Autodesk Fusion 360 part; units mm, degrees
sketch "Sketch1" plane through (0, 0, 0) normal (0, 0, 1) x (1, 0, 0)
  line L0 (-26.35, 10.5) -> (-26.35, -10.5)
  line L1 (-26.35, -10.5) -> (-16.35, -10.5)
  line L2 (-16.35, -10.5) -> (-16.35, 10.5)
  line L3 (-16.35, 10.5) -> (16.35, 10.5)
  line L4 (16.35, 10.5) -> (16.35, -10.5)
  line L5 (16.35, -10.5) -> (26.35, -10.5)
  line L6 (26.35, -10.5) -> (26.35, 10.5)
  line L7 (-26.35, -10.5) -> (26.35, 10.5) construction
  line L8 (-26.35, 10.5) -> (-26.35, 31)
  line L9 (-26.35, 31) -> (26.35, 31)
  line L10 (26.35, 31) -> (26.35, 10.5)
  line L11 (-22.75, 31) -> (22.75, 31) construction
  line L12 (22.75, 31) -> (22.75, 10.5) construction
  line L13 (22.75, 10.5) -> (-22.75, 10.5) construction
  line L14 (-22.75, 10.5) -> (-22.75, 31) construction
  line L15 (-22.75, 10.5) -> (22.75, 31) construction
  circle A0 centre (-21.35, 11.9) radius 0.975
  line L16 (-22.75, 20.75) -> (22.75, 20.75) construction
  line L17 (0, 10.5) -> (0, 31) construction
  circle A1 centre (-21.35, 29.6) radius 0.975
  circle A2 centre (21.35, 11.9) radius 0.975
  circle A3 centre (21.35, 29.6) radius 0.975
  circle A4 centre (-12.75, 20.75) radius 8.05
  circle A5 centre (12.75, 20.75) radius 8.05
  line L18 (0, 10.5) -> (0, 31) construction
  line L19 (5.5, 31) -> (5.5, 25.5)
  line L20 (5.5, 25.5) -> (-5.5, 25.5)
  line L21 (-5.5, 25.5) -> (-5.5, 31)
  line L22 (5, 14.5) -> (-5, 14.5)
  line L23 (-5, 14.5) -> (-5, 10.5)
  line L24 (5, 10.5) -> (5, 14.5)
  point P0 (0, 20.75)
  point P1 (0, 20.75)
  point P2 (0, 31.5)
  point P3 (0, 25.5)
  point P4 (0, 14.5)
  dimension "d3" = 10
  dimension "d4" = 52.7
  dimension "d5" = 21
  dimension "d6" = 20.5
  dimension "d7" = 45.5
  dimension "d8" = 20.5
  dimension "d9" = 1.95
  dimension "d10" = 1.4
  dimension "d11" = 1.4
  dimension "d12" = 16.1
  dimension "d13" = 10
  dimension "d16" = 11
  dimension "d17" = 5.5
  dimension "d19" = 4
  dimension "d20" = 10
extrude "Extrude1" add sketch "Sketch1" along normal blind 3 contours L0 L1 L2 L3 L4 L5 L6 L8 L9 L10 L19 L20 L21 L22 L23 L24
sketch "Sketch2" plane through (0, -10.5, 0) normal (0, -1, 0) x (1, 0, 0)
  line L0 (16.35, 0) -> (26.35, 0)
  line L1 (26.35, 0) -> (26.35, 3)
  line L2 (26.35, 3) -> (16.35, 3)
  line L3 (16.35, 3) -> (16.35, 0)
  line L4 (16.35, 0) -> (16.35, -5)
  line L5 (16.35, -5) -> (26.35, -5)
  line L6 (26.35, -5) -> (26.35, 0)
  line L7 (0, 0) -> (0, -5) construction
  line L8 (-16.35, 0) -> (-16.35, -5)
  line L9 (-16.35, -5) -> (-26.35, -5)
  line L10 (-26.35, -5) -> (-26.35, 0)
  line L11 (-26.35, 0) -> (-16.35, 0)
  circle A0 centre (21.35, -2.5) radius 1.5
  line L12 (16.35, 0) -> (26.35, -5) construction
  circle A1 centre (-21.35, -2.5) radius 1.5
  dimension "d21" = 5
  dimension "d24" = 3
extrude "Extrude2" add sketch "Sketch2" against normal blind 3 contours L0 L4 L5 L6 | L8 L9 L10 L11
sketch "Sketch3" plane through (26.35, 0, 0) normal (1, 0, 0) x (0, 0, -1)
  line L0 (0, -7.5) -> (0, 31)
  line L1 (0, 31) -> (-3, 31)
  line L2 (-3, 31) -> (-3, -10.5)
  line L3 (-3, -10.5) -> (5, -10.5)
  line L4 (5, -10.5) -> (5, -7.5)
  line L5 (5, -7.5) -> (0, -7.5)
  line L6 (5, -7.5) -> (0, 1.1603)
  line L7 (0, 1.1603) -> (0, -7.5)
  line L8 (5, -7.5) -> (0, -7.5)
  dimension "d27" = 60
extrude "Extrude3" add sketch "Sketch3" against normal blind 1.5 contours L0 L5 L6 L7 L8
extrude "Extrude4" add sketch "Sketch3" along normal blind 1.5 from surface at -10 contours L0 L5 L6 L7 L8
extrude "Extrude5" add sketch "Sketch3" along normal blind 1.5 from surface at -52.7 contours L0 L5 L6 L7 L8
extrude "Extrude6" add sketch "Sketch3" against normal blind 1.5 from surface at -42.7 contours L0 L5 L6 L7 L8
chamfer "Chamfer1" distance 2 angle 45 8 edges at (26.35, -10.5, -1) (16.35, -10.5, -1) (-16.35, -10.5, -1) (-26.35, -10.5, -1) (-5, 14.5, 1.5) (5, 14.5, 1.5) (5, 10.5, 1.5) (-5, 10.5, 1.5)
chamfer "Chamfer1" distance 4 angle 45 4 edges at (-16.35, 10.5, 1.5) (16.35, 10.5, 1.5) (26.35, 31, 1.5) (-26.35, 31, 1.5)
chamfer "Chamfer1" distance 0.5 angle 45 6 edges at (5.2448, 23.661, 3) (5.2448, 23.661, 0) (-20.2552, 23.661, 3) (-20.2552, 23.661, 0) (-5.5, 25.5, 1.5) (5.5, 25.5, 1.5)
chamfer "Chamfer1" distance 4 angle 45 2 edges at (-5.5, 31, 1.5) (5.5, 31, 1.5)
Source: CAD feature listing. Evaluate the final solid. Frame: model axes, mm. A direction names the side the tool comes from. Coordinates: 2 decimals unless noted, no trailing zeros. Loops run counter-clockwise (first coordinate to the right, second up) from the corner with the lowest first, then second, coordinate; pieces in that order, holes last. Notation, with made-up numbers: (64.5, 65) -> (91.5, 65) arc R8 cw to (91.5, 76) -> close; hole circle Ø2 at (-36, 10.5). An arc over 180 degrees is marked (long way). One line per item, written item: value. Start each with the question number.
Q1. Mould query, pull axis Y, two halves, no side actions, for faces 4 (the face through (19.7, -7.5, -2.5)), 5 (the face through (-21.561, 12.852, 1.479)), 6 (the face through (-16.35, -3, 0)). Classes: pulls with the +Y half, pulls with the -Y half, needs draft (parallel to the pull), parting line crosses it, or undercut.
Q2. Section query C-C, the plane y = -4.5. Return the cut outline in (x, z).
Q3. Contact query for flat-ended pins moving along their axis: P1, Ø3, axis at x = -21.35, y = 29.6, coming from the +Z side; P2, Ø3, axis at y = 20.5, z = -2.5, coming from the -X side; P3, Ø1.5, axis at x = 22.5, z = -1.5, coming from the +Y side; P4, Ø12, axis at x = -9.5, y = 18.5, coming from the -Z side. Output: stop coordinate, or through.
Q4. Section query B-B, the plane z = -2.5. Return the cut outline in (x, y).
Q5. Section query D-D, the plane x = 2. Return the cut outline in (y, z), and give its area (3 significant figures).
Q6. Set-up query: faces 1 (the face through (-17.85, -5, -1)), 2 (the face through (-4, 13.5, 1.5)), 3 (the face through (0, 15, 3)). Return all of +Z, -Z, +X, -X, +Y, -Y with unobstructed straight access to the full face (end or side cutting, diameter ignored); none if empty.
Q7. Section query A-A, the plane y = 4. Return the cut outline in (x, z).
Q8. Line query: line 1 along Y through (x, z) = (21.35, 2.2) (3 decimals); line 2 along X through (y, z) = (17, 1.25); line 3 along X through (y, z) = (-6, 2.5). Output: solid intervals per line, ascending.
Results:
1. face 4: pulls with the +Y half
1. face 5: undercut
1. face 6: needs draft
2. outline: (-26.35, -3.27) -> (-24.85, -3.27) -> (-24.85, 0) -> (-17.85, 0) -> (-17.85, -3.27) -> (-16.35, -3.27) -> (-16.35, 3) -> (-26.35, 3) -> close; (16.35, -3.27) -> (17.85, -3.27) -> (17.85, 0) -> (24.85, 0) -> (24.85, -3.27) -> (26.35, -3.27) -> (26.35, 3) -> (16.35, 3) -> close
3. P1: z = 3
3. P2: through
3. P3: y = -7.5
3. P4: z = 0
4. outline: (-26.35, -8.5) -> (-24.35, -10.5) -> (-22.85, -10.5) -> (-22.85, -7.5) -> (-24.85, -7.5) -> (-24.85, -3.17) -> (-26.35, -3.17) -> close; (-19.85, -10.5) -> (-18.35, -10.5) -> (-16.35, -8.5) -> (-16.35, -3.17) -> (-17.85, -3.17) -> (-17.85, -7.5) -> (-19.85, -7.5) -> close; (16.35, -8.5) -> (18.35, -10.5) -> (19.85, -10.5) -> (19.85, -7.5) -> (17.85, -7.5) -> (17.85, -3.17) -> (16.35, -3.17) -> close; (22.85, -10.5) -> (24.35, -10.5) -> (26.35, -8.5) -> (26.35, -3.17) -> (24.85, -3.17) -> (24.85, -7.5) -> (22.85, -7.5) -> close
5. outline: (14.5, 0) -> (25.5, 0) -> (25.5, 3) -> (14.5, 3) -> close
5. area: 33.0 mm^2
6. face 1: -Z, +Y
6. face 2: +Z, -Z, -Y
6. face 3: +Z, +X, -X, +Y, -Y
7. outline: (-26.35, 0) -> (-16.35, 0) -> (-16.35, 3) -> (-26.35, 3) -> close; (16.35, 0) -> (26.35, 0) -> (26.35, 3) -> (16.35, 3) -> close
8. line 1: -10.5 to 10.925, 12.875 to 28.625, 30.575 to 31
8. line 2: -26.35 to -19.87, -5.63 to 5.63, 19.87 to 26.35
8. line 3: -26.35 to -16.35, 16.35 to 26.35
